CAD build for the part. Positions are in the model's coordinates, mm. Face numbers are marked on the shaded views. A direction names the side the tool comes from. Give positions to 0.01 mm unless a question says otherwise; leave off trailing zeros. Loops run counter-clockwise (first coordinate to the right, second up) from the corner with the lowest first, then second, coordinate; pieces in that order, holes last. Notation, with made-up numbers: (52, 30) - (95, 30) arc R32 cw to (95, 56) - close; hole circle Ø2 at (7, 39). An arc over 180 degrees is marked (long way). Return JSON: item names as keys, results as strings.
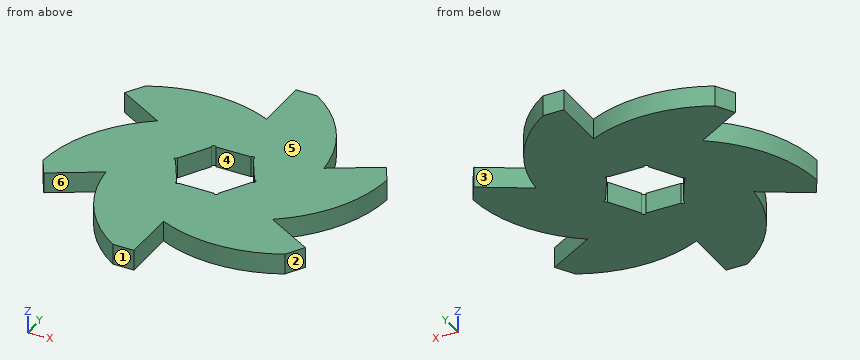
from build123d import *

# Parameters (mm, degrees)
BOSS_EXTRUDE1_DEPTH = 15


with BuildPart() as part:
    # Sketch1 → Boss-Extrude1 (new body)
    with BuildSketch(Plane.XY):
        with BuildLine():
            Line((0, 70), (0, 110))
            Line((0, 110), (15.459491817, 110))
            ThreePointArc((15.459491817, 110), (46.684314733, 77.704911176), (60.621778265, 35))
            Line((60.621778265, 35), (95.262794416, 55))
            Line((95.262794416, 55), (102.992540325, 41.611687357))
            ThreePointArc((102.992540325, 41.611687357), (90.636584443, -1.577346929), (60.621778265, -35))
            Line((60.621778265, -35), (95.262794416, -55))
            Line((95.262794416, -55), (87.533048508, -68.388312643))
            ThreePointArc((87.533048508, -68.388312643), (43.952269711, -79.282258105), (0, -70))
            Line((0, -70), (0, -110))
            Line((0, -110), (-15.459491817, -110))
            ThreePointArc((-15.459491817, -110), (-46.684314733, -77.704911176), (-60.621778265, -35))
            Line((-60.621778265, -35), (-95.262794416, -55))
            Line((-95.262794416, -55), (-102.992540325, -41.611687357))
            ThreePointArc((-102.992540325, -41.611687357), (-90.636584443, 1.577346929), (-60.621778265, 35))
            Line((-60.621778265, 35), (-95.262794416, 55))
            Line((-95.262794416, 55), (-87.533048508, 68.388312643))
            ThreePointArc((-87.533048508, 68.388312643), (-43.952269711, 79.282258105), (0, 70))
        make_face()
        with BuildLine():
            Line((-28.003972595, -1.495696651), (-15.297297594, -23.504303349))
            ThreePointArc((-15.297297594, -23.504303349), (-14.80875673, -25.649519053), (-12.706675001, -25))
            Line((-12.706675001, -25), (12.706675001, -25))
            ThreePointArc((12.706675001, -25), (14.80875673, -25.649519053), (15.297297594, -23.504303349))
            Line((15.297297594, -23.504303349), (28.003972595, -1.495696651))
            ThreePointArc((28.003972595, -1.495696651), (29.617513459, 0), (28.003972595, 1.495696651))
            Line((28.003972595, 1.495696651), (15.297297594, 23.504303349))
            ThreePointArc((15.297297594, 23.504303349), (14.80875673, 25.649519053), (12.706675001, 25))
            Line((12.706675001, 25), (-12.706675001, 25))
            ThreePointArc((-12.706675001, 25), (-14.80875673, 25.649519053), (-15.297297594, 23.504303349))
            Line((-15.297297594, 23.504303349), (-28.003972595, 1.495696651))
            ThreePointArc((-28.003972595, 1.495696651), (-29.617513459, 0), (-28.003972595, -1.495696651))
        make_face(mode=Mode.SUBTRACT)
    extrude(amount=BOSS_EXTRUDE1_DEPTH)


solid = part.part
1. Drill centre lines: probe 1 along Y at (x, z) = (-68.5, 5); probe 2 along X at (y, z) = (13.5, 10.25); probe 3 along X at (y, z) = (-5.5, 14). Where is each one in solid material? Low to high.
Values follow:
{"probe 1": "y = -39.55 to 28.85, 39.55 to 75.75", "probe 2": "x = -82.89 to -21.07, 21.07 to 97.41", "probe 3": "x = -94.19 to -25.69, 25.69 to 88.35"}
2. Cut at D-D, the plane y = 87. Write the cut outline in (x, z), plus the area to 3 significant figures.
Values follow:
{"outline": "(0, 0) - (40.35, 0) - (40.35, 15) - (0, 15) - close", "area": "605 mm²"}
3. Drop flat-ended pins along their axis: P1, Ø6, axis at x = 13, z = 5, coming from the -Y side; P2, Ø5, axis at y = -41.5, z = 12.5, coming from the +X side; P3, Ø3, axis at x = -66, z = 12.5, coming from the -Y side. Give the stop position or say it passes through.
Values follow:
{"P1": "stops at y = -75.83", "P2": "stops at x = 76.21", "P3": "stops at y = -38.97"}
4. Cut at C-C, the plane x = 25. Write the cut outline in (y, z), plus the area to 3 significant figures.
Values follow:
{"outline": "(-77.82, 0) - (-6.7, 0) - (-6.7, 15) - (-77.82, 15) - close; (6.7, 0) - (102.97, 0) - (102.97, 15) - (6.7, 15) - close", "area": "2,510 mm²"}
5. Pull direction X, two halves, no side cores. Call the marked faces 1, 2 and 3: +X half, -X half, draft (parallel to the pull), parting line (faces both ways), or undercut.
Values follow:
{"face 1": "draft", "face 2": "+X half", "face 3": "undercut"}
6. Which spindle directions (+Z, -Z, +X, -X, +Y, -Y) get a long thin tool onto all of the face, cutting with end or side? Do the marked faces 4, 5 and 6. Say none if no direction does.
Values follow:
{"face 4": "+Z, -Z", "face 5": "+Z, +X, -X, +Y, -Y", "face 6": "+Z, -Z, -Y"}
7. Cut at A-A, the plane y = 49.5. Write the cut outline in (x, z), plus the area to 3 significant figures.
Values follow:
{"outline": "(-85.74, 0) - (58.25, 0) - (58.25, 15) - (-85.74, 15) - close; (85.74, 0) - (98.44, 0) - (98.44, 15) - (85.74, 15) - close", "area": "2,350 mm²"}
